from build123d import *

# Parameters (mm, degrees)
BOSS_EXTRUDE1_DEPTH = 6
BOSS_EXTRUDE2_DEPTH = 40


with BuildPart() as part:
    # Sketch2 → Boss-Extrude1 (new body)
    with BuildSketch(Plane(origin=(0, 0, 0), x_dir=(1, 0, 0), z_dir=(0, 1, 0))):
        with BuildLine():
            Line((-290.127976468, -122.862929175), (397.464433619, -122.862929175))
            ThreePointArc((397.464433619, -122.862929175), (478.668228576, -41.659134218), (397.464433619, 39.544660738))
            Line((397.464433619, 39.544660738), (-290.127976468, 39.544660738))
            ThreePointArc((-290.127976468, 39.544660738), (-371.331771424, -41.659134218), (-290.127976468, -122.862929175))
        make_face()
    extrude(amount=BOSS_EXTRUDE1_DEPTH)

    # Sketch2_3 → Boss-Extrude2 (add)
    with BuildSketch(Plane(origin=(0, 0, 0), x_dir=(1, 0, 0), z_dir=(0, 1, 0))):
        with BuildLine():
            ThreePointArc((-370.713684353, -51.659134218), (-371.331771424, -41.659134218), (-370.713684353, -31.659134218))
            Line((-370.713684353, -31.659134218), (-421.331771424, -31.659134218))
            Line((-421.331771424, -31.659134218), (-421.331771424, -51.659134218))
            Line((-421.331771424, -51.659134218), (-370.713684353, -51.659134218))
        make_face()
        with BuildLine():
            Line((528.668228576, -31.659134214), (478.050141504, -31.659134214))
            ThreePointArc((478.050141504, -31.659134214), (478.668228576, -41.659134214), (478.050141505, -51.659134214))
            Line((478.050141505, -51.659134214), (528.668228576, -51.659134214))
            Line((528.668228576, -51.659134214), (528.668228576, -31.659134214))
        make_face()
    extrude(amount=BOSS_EXTRUDE2_DEPTH)


solid = part.part
Design review of the part built by this model. Coordinates are the model's own, in mm. A direction names the side the tool comes from. Round coordinates to 2 decimals unless told otherwise and drop trailing zeros. Write each loop counter-clockwise with the first axis right and the second up, starting at its lowest first coordinate (ties: lowest second). Pieces come first, ordered by that corner, then holes. Notation, with made-up numbers: (18.25, -7.5) - (38.25, -7.5) arc R21 cw to (38.25, 15.5) - close; hole circle Ø7 at (87.5, 49). An arc over 180 degrees is marked (long way). Use a Markdown table: item, result. Add a question column.
1. Mouldability with a two-part tool opening along X and no side actions: class faces 3 (the face through (450.613, 2.958, 103.053)), 4 (the face through (-396, 40, 42)), 5 (the face through (-371.33, 22.76, 41.8)), 6 (the face through (-343.277, 2.958, -19.735)) as +X half, -X half, draft (parallel to the pull), parting line (faces both ways), or undercut.
2. We need section B-B (z = 43). State the section outline as (x, y) points.
3. We need section D-D (z = 102). State the section outline as (x, y) points, then the cut area to 3 significant figures.
4. Wall thickness on probe 1 along X at (y, z) = (14, 37.5); probe 2 along Y at (x, z) = (461.5, 39.5); probe 3 along X at (y, z) = (26, 35.5): over which ranges is each line inside the solid? List them lowest first.
5. Clearance check with flat-ended pins moving along their axes: pin 1 (20 mm diameter, centred on x = 493, y = 26.5, fed in from -Z); pin 2 (3 mm diameter, centred on x = 154.5, z = 0.5, fed in from +Y). State where each tip first meets the part, or that it passes through.
6. We need section A-A (y = 16). State the section outline as (x, z) points, then the cut area to 3 significant figures.
7. For faces 1 (the face through (-421.332, 20, 42)), 2 (the face through (478.67, 22.76, 41.52)), list the 3-axis set-ups (+Z, -Z, +X, -X, +Y, -Y) from which the entire face can be reached by the end or side of a thin tool; tool diameter is ignored.
8. We need section C-C (x = 53.5). State the section outline as (y, z) points.
Output:
| question | item | result |
|---|---|---|
| 1 | face 3 | +X half |
| 1 | face 4 | draft |
| 1 | face 5 | undercut |
| 1 | face 6 | -X half |
| 2 | outline | (-421.33, 0) - (528.67, 0) - (528.67, 40) - (478.66, 40) - (478.66, 6) - (-371.32, 6) - (-371.32, 40) - (-421.33, 40) - close |
| 3 | outline | (-344.47, 0) - (451.81, 0) - (451.81, 6) - (-344.47, 6) - close |
| 3 | area | 4,780 mm2 |
| 4 | probe 1 | x = -421.33 to -371.23, 478.56 to 528.67 |
| 4 | probe 2 | y = 0 to 6 |
| 4 | probe 3 | x = -421.33 to -371.1, 478.43 to 528.67 |
| 5 | pin 1 | stops at z = 31.66 |
| 5 | pin 2 | stops at y = 6 |
| 6 | outline | (-421.33, 31.66) - (-370.71, 31.66) arc R81.2 cw to (-370.71, 51.66) - (-421.33, 51.66) - close; (478.05, 31.66) - (528.67, 31.66) - (528.67, 51.66) - (478.05, 51.66) arc R81.2 cw to start |
| 6 | area | 2,010 mm2 |
| 7 | face 1 | +Z, -Z, -X, +Y, -Y |
| 7 | face 2 | +Y |
| 8 | outline | (0, -39.54) - (6, -39.54) - (6, 122.86) - (0, 122.86) - close |
